Read the model definition and answer for the solid it produces. Units are mm, in the model's axes. A direction names the side the tool comes from. Round coordinates to 2 decimals unless told otherwise and drop trailing zeros. Order: outer loops, then holes, each group sorted by start corner. A loop starts at its lowest first (then second) coordinate and runs counter-clockwise, first axis right, second up. Notation, with made-up numbers: (75, 13.5) - (129, 13.5) arc R9 cw to (129, 20.5) - close; hole circle Ø11 at (25.5, -11.75). An arc over 180 degrees is marked (long way). Answer as a JSON object with one key per item and string values. Group by question number.
Q1. A cutting plane is placed at C-C on y = 258. Determine the outline of the cut face in (x, z).
Q2. Consider line 1 (Z direction, x = 0.5, y = 201); line 2 (X direction, y = 193.5, z = -9.5); line 3 (Y direction, x = -11.5, z = 10.5). Determine where each line is inside the solid, lowest interval first.
Q3. A cutting plane is placed at B-B on z = 6.5. Determine the outline of the cut face in (x, y).
Q4. The mould has two halves that part along X. Classify faces 1 (the flat face through (12.7, 301, 0)), 2 (the flat face through (-12.7, 301, 0)), 3 (the flat face through (0, 301, -23.812)): pulls with the +X half, pulls with the -X half, needs draft (parallel to the pull), parting line crosses it, or undercut.
Q5. A cutting plane is placed at A-A on x = -6. Determine the outline of the cut face in (y, z), and give its area (3 significant figures).
Q6. A tool of negligible diameter and unlimited length cuts with its end or side. For faces 4 (the flat face through (0, 301, 23.812)), 5 (the flat face through (0, 301, -25.4)), from which of +Z, -Z, +X, -X, +Y, -Y can it reach the whole face along a straight path? Write none if from no direction.
```python
from build123d import *

# Parameters (mm, degrees)
SKETCH1_W               = 25.4
SKETCH1_H               = 50.8
SKETCH1_W_2             = 22.225
SKETCH1_H_2             = 47.625
BOSS_EXTRUDE1_DEPTH     = 609.6
CUT_EXTRUDE1_DEPTH      = 611.657416233
CUT_EXTRUDE2_DEPTH      = 611.261099858
CUT_EXTRUDE2_DEPTH_BACK = 611.261099858


with BuildPart() as part:
    # Sketch1 → Boss-Extrude1 (new body)
    with BuildSketch(Plane(origin=(0, 0, 0), x_dir=(1, 0, 0), z_dir=(0, 1, 0))):
        Rectangle(SKETCH1_W, SKETCH1_H)
        Rectangle(SKETCH1_W_2, SKETCH1_H_2, mode=Mode.SUBTRACT)
    extrude(amount=BOSS_EXTRUDE1_DEPTH)

    # Sketch2 → Cut-Extrude1 (cut, through all)
    with BuildSketch(Plane(origin=(12.7, 0, 0), x_dir=(0, 0, -1), z_dir=(1, 0, 0))):
        Polygon((25.4, 609.6), (-25.4, 609.6), (-25.4, 580.270606325), align=None)
    extrude(amount=-CUT_EXTRUDE1_DEPTH, mode=Mode.SUBTRACT)

    # Sketch3 → Cut-Extrude2 (cut, two sides: drawn at the far end of the back side and taken through both)
    with BuildSketch(Plane(origin=(0, 0, 0), x_dir=(0, 0, -1), z_dir=(1, 0, 0)).offset(-CUT_EXTRUDE2_DEPTH_BACK)):
        Polygon((-25.4, 0), (25.4, 0), (-25.4, 29.329393675), align=None)
    extrude(amount=CUT_EXTRUDE2_DEPTH + CUT_EXTRUDE2_DEPTH_BACK, mode=Mode.SUBTRACT)


solid = part.part
```
Result set:
{
 "1": {"outline": "(-12.7, -25.4) - (12.7, -25.4) - (12.7, 25.4) - (-12.7, 25.4) - close; hole (-11.11, -23.81) - (11.11, -23.81) - (11.11, 23.81) - (-11.11, 23.81) - close"},
 "2": {"line 1": "z = -25.4 to -23.81, 23.81 to 25.4", "line 2": "x = -12.7 to -11.11, 11.11 to 12.7", "line 3": "y = 20.73 to 588.87"},
 "3": {"outline": "(-12.7, 18.42) - (-11.11, 18.42) - (-11.11, 591.18) - (-12.7, 591.18) - close; (11.11, 18.42) - (12.7, 18.42) - (12.7, 591.18) - (11.11, 591.18) - close"},
 "4": {"face 1": "pulls with the +X half", "face 2": "pulls with the -X half", "face 3": "undercut"},
 "5": {"outline": "(0, -25.4) - (609.6, -25.4) - (608.68, -23.81) - (0.92, -23.81) - close; (28.41, 23.81) - (581.19, 23.81) - (580.27, 25.4) - (29.33, 25.4) - close", "area": "1,840 mm²"},
 "6": {"face 4": "+Y, -Y", "face 5": "-Z, +X, -X, +Y, -Y"}
}
